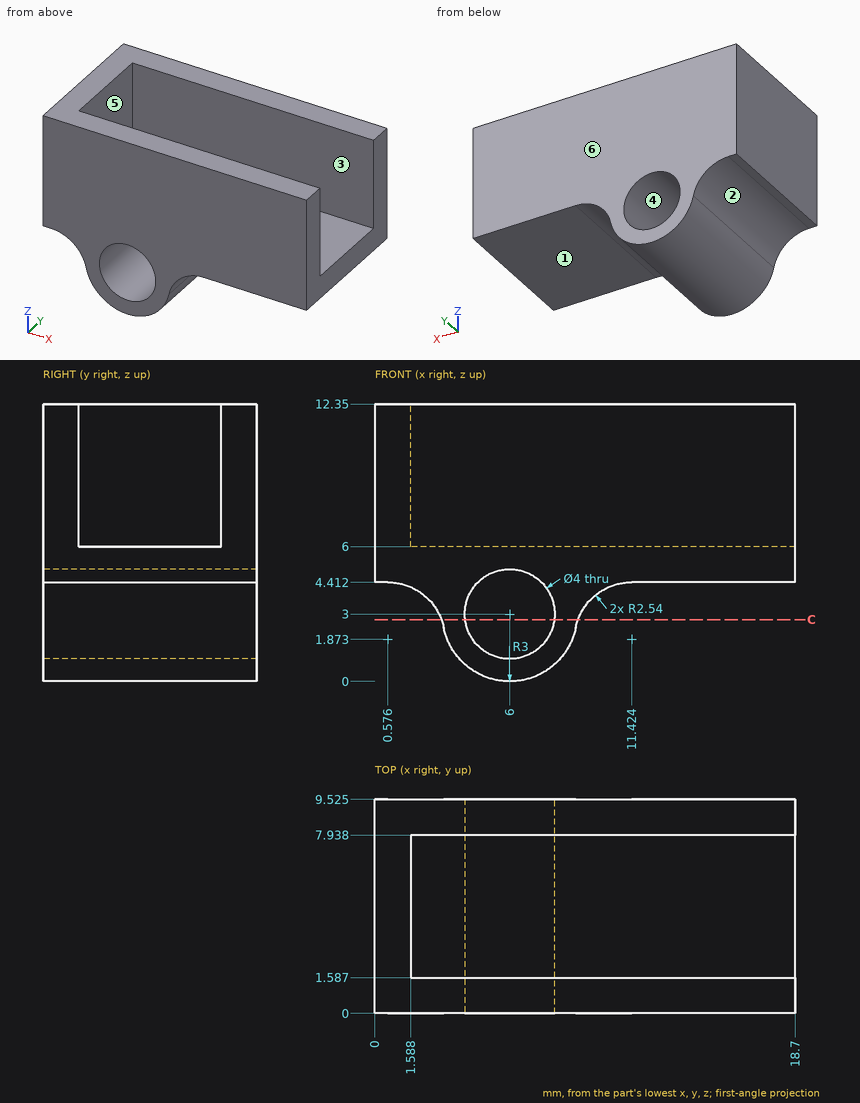
Design review of the part shown in the three views and the two pictorial views. Dimensions are in mm from the part's minimum x, y and z. A direction names the side the tool comes from. Give positions to 0.01 mm unless a question says otherwise; leave off trailing zeros. Write each loop counter-clockwise with the first axis right and the second up, starting at its lowest first coordinate (ties: lowest second). Pieces come first, ordered by that corner, then holes.
Item 1: Insertion check: P1, Ø1, axis at y = 1.5, z = 10.5, coming from the -X side; P2, Ø1.5, axis at y = 4, z = 7.5, coming from the +X side; P3, Ø5, axis at x = 7, y = 4.5, coming from the +Z side. Each pin has a flat end and moves straight along its axis. Give the tip position at first contact, or say it passes through.
Item 2: Wall thickness on probe 1 along Y at (x, z) = (8.75, 11.25) (1 decimal); probe 2 along X at (y, z) = (6.5, 7); probe 3 along X at (y, z) = (5, 1.75) (1 decimal): over which ranges is each line inside the solid? List them lowest first.
Item 3: Take a section at C-C (z = 2.75). Give the boundary of the cut face in (x, y) (1 decimal).
Item 4: Machinability: for the marked faces 1, 2 and 3, which of the approach directions +Z, -Z, +X, -X, +Y, -Y give a long, thin tool a straight path to every point of the face, cutting with its end or side? Answer none if there is none.
Item 5: The part is to be moulded in two halves that separate along Y. For the marked faces 4, 5 and 6, say which applies: +Y half, -Y half, draft (parallel to the pull), parting line (faces both ways), or undercut.
Established:
1. P1: stops at x = 0
1. P2: stops at x = 1.59
1. P3: stops at z = 6
2. probe 1: y = 0 to 1.6, 7.9 to 9.5
2. probe 2: x = 0 to 1.59
2. probe 3: x = 3.3 to 4.4, 7.6 to 8.7
3. outline: (3, 0) - (4, 0) - (4, 9.5) - (3, 9.5) - close; (8, 0) - (9, 0) - (9, 9.5) - (8, 9.5) - close
4. face 1: -Z, +X, +Y, -Y
4. face 2: -Z, -X, +Y, -Y
4. face 3: +Z, +X
5. face 4: draft
5. face 5: undercut
5. face 6: +Y half
